For this review, take the finished solid that the model builds, in its own axes (mm). Face numbers are marked on the shaded views. A direction names the side the tool comes from. Coordinates: 2 decimals unless noted, no trailing zeros. Order: outer loops, then holes, each group sorted by start corner. A loop starts at its lowest first (then second) coordinate and runs counter-clockwise, first axis right, second up.
from build123d import *

# Parameters (mm, degrees)
F1_DEPTH       = 2
F2_W           = 50.8
F2_H           = 50.8
F2_W_2         = 46.8
F2_H_2         = 46.8
F3_DEPTH       = 8.89
F4_R           = 3.127246
F5_DEPTH       = 25.4
F6_W           = 25.4
F6_H           = 2
F7_DEPTH       = 25.4
F8_W           = 50.8
F8_H           = 50.8
F9_DEPTH       = 1
F10_W          = 1
F10_H          = 25.4
F11_DEPTH      = 1
F12_W          = 10
F12_H          = 2
F13_DEPTH      = 1
F13_DEPTH_BACK = 0.1


with BuildPart() as f1:
    # F0 (on Top) → F1 (new body)
    with BuildSketch(Plane.XY):
        Polygon((50.8, 25.4), (-50.8, 25.4), (-50.8, -25.4), (50.8, -25.4), (50.8, -12.7), (14.7, -12.7), (14.7, 12.7), (50.8, 12.7), align=None)
    extrude(amount=F1_DEPTH)

    # F2 (on face) → F3 (join)
    with BuildSketch(Plane.XY.offset(2)):
        with Locations((25.4, 0)):
            Rectangle(F2_W, F2_H)
        with Locations((25.4, 0)):
            Rectangle(F2_W_2, F2_H_2, mode=Mode.SUBTRACT)
    extrude(amount=F3_DEPTH)

    # F4 (on face) → F5 (cut)
    with BuildSketch(Plane(origin=(0, 0, 0), x_dir=(0, -1, 0), z_dir=(-1, 0, 0))):
        with Locations((-1.785935, 6.089438)):
            Circle(F4_R)
    extrude(amount=-F5_DEPTH, mode=Mode.SUBTRACT)

    # F6 (on face) → F7 (cut)
    with BuildSketch(Plane.YZ.offset(50.8)):
        with Locations((0, 3)):
            Rectangle(F6_W, F6_H)
    extrude(amount=-F7_DEPTH, mode=Mode.SUBTRACT)

    # F8 (on face) → F9 (cut)
    with BuildSketch(Plane.XY.offset(10.89)):
        with Locations((25.4, 0)):
            Rectangle(F8_W, F8_H)
    extrude(amount=-F9_DEPTH, mode=Mode.SUBTRACT)

    # F10 (on face) → F11 (cut)
    with BuildSketch(Plane.XY.offset(2)):
        with Locations((13.2, 0)):
            Rectangle(F10_W, F10_H)
    extrude(amount=-F11_DEPTH, mode=Mode.SUBTRACT)

    # F12 (on face) → F13 (join, two sides)
    with BuildSketch(Plane.XY.offset(2)) as f13_sk:
        with Locations((19.7, -12.7)):
            Rectangle(F12_W, F12_H)
        with Locations((19.7, 12.7)):
            Rectangle(F12_W, F12_H)
    extrude(amount=F13_DEPTH)
    extrude(f13_sk.sketch, amount=-F13_DEPTH_BACK)


solid = f1.part
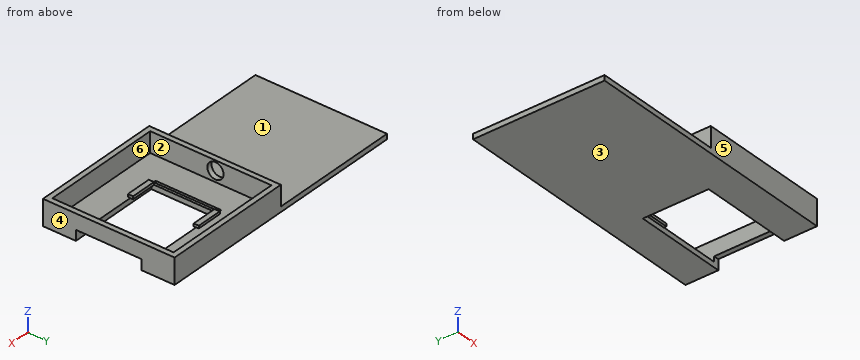
1. Take a section at D-D, the plane z = 7.75. Give the boundary of the cut face in (x, y).
Answer below:
outline: (0, -25.4) - (50.8, -25.4) - (50.8, 25.4) - (0, 25.4) - (0, 4.44) - (2, 4.44) - (2, 23.4) - (48.8, 23.4) - (48.8, -23.4) - (2, -23.4) - (2, -0.86) - (0, -0.86) - close
2. Take a section at B-B, the plane y = 6. Give the boundary of the cut face in (x, z), plus the area to 3 significant figures.
Answer below:
outline: (-50.8, 0) - (14.7, 0) - (14.7, 2) - (13.7, 2) - (13.7, 1) - (12.7, 1) - (12.7, 2) - (2, 2) - (2, 9.89) - (0, 9.89) - (0, 2) - (-50.8, 2) - close; (48.8, 4) - (50.8, 4) - (50.8, 9.89) - (48.8, 9.89) - close
area: 158 mm2
3. Take a section at A-A, the plane x = 45. Give the boundary of the cut face in (y, z).
Answer below:
outline: (-25.4, 0) - (-12.7, 0) - (-12.7, 2) - (-23.4, 2) - (-23.4, 9.89) - (-25.4, 9.89) - close; (12.7, 0) - (25.4, 0) - (25.4, 9.89) - (23.4, 9.89) - (23.4, 2) - (12.7, 2) - close
4. Clearance check with flat-ended pins moving along their axes: pin 1 Ø1.6 at (y, z) = (4.5, 1) entering from +X; pin 2 Ø5 at (y, z) = (1, 7.5) entering from -X; pin 3 Ø1 at (x, y) = (-6, -1) entering from +Z. State where each tip first meets the part, or that it passes through.
Answer below:
pin 1: stops at x = 14.7
pin 2: stops at x = 0
pin 3: stops at z = 2
5. Take a section at C-C, the plane y = 22. Give the boundary of the cut face in (x, z).
Answer below:
outline: (-50.8, 0) - (50.8, 0) - (50.8, 9.89) - (48.8, 9.89) - (48.8, 2) - (2, 2) - (2, 9.89) - (0, 9.89) - (0, 2) - (-50.8, 2) - close
6. To check wall thickness, follow L1, parallel to X at y = -3.5, z = 7; L2, parallel to Y at x = 11.5, z = 6.5; L3, parallel to Z at x = -26, y = -4. State the ranges of each line that lie inside material, in increasing order.
Answer below:
L1: x = 0 to 2, 48.8 to 50.8
L2: y = -25.4 to -23.4, 23.4 to 25.4
L3: z = 0 to 2
7. Machinability: for the marked faces 1, 2 and 3, which of the approach directions +Z, -Z, +X, -X, +Y, -Y give a long, thin tool a straight path to every point of the face, cutting with its end or side? Answer none if there is none.
Answer below:
face 1: +Z, -X, +Y, -Y
face 2: +Z
face 3: -Z, +X, -X, +Y, -Y
8. The part is to be moulded in two halves that separate along X. For the marked faces 4, 5 and 6, say which applies: +X half, -X half, draft (parallel to the pull), parting line (faces both ways), or undercut.
Answer below:
face 4: +X half
face 5: draft
face 6: undercut
